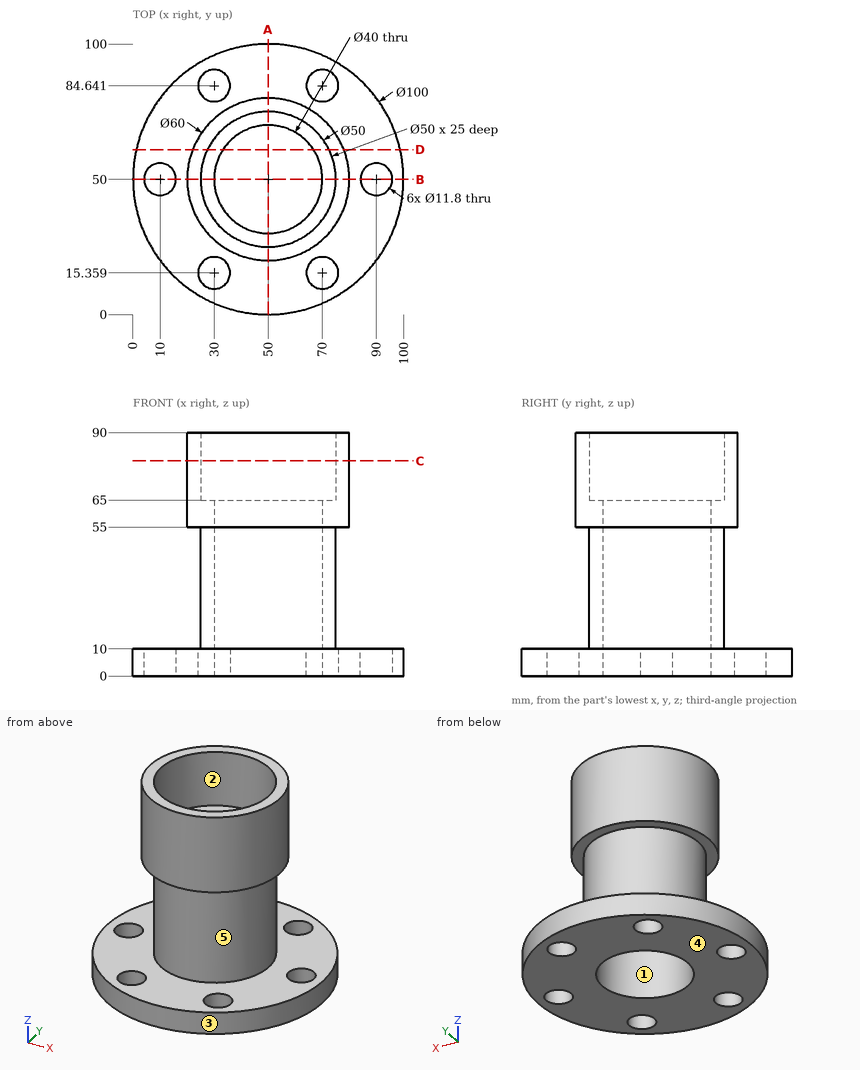
Here's the drawing with two shaded views (mm, measured from the low corner). I have some questions. A direction names the side the tool comes from. Give positions to 0.01 mm unless a question says otherwise; leave off trailing zeros. Loops run counter-clockwise (first coordinate to the right, second up) from the corner with the lowest first, then second, coordinate; pieces in that order, holes last. Notation, with made-up numbers: (72, 10.5) -> (96, 10.5) arc R21 ccw to (96, 32.5) -> close; hole circle Ø6 at (55, 2). An arc over 180 degrees is marked (long way). One line per item, written item: value.
Q1. We'd pull the mould along Z, two halves only. Please class the marked faces 3, 4 and 5: pulls with the +Z half, pulls with the -Z half, needs draft (parallel to the pull), parting line crosses it, or undercut.
Answers follow:
face 3: needs draft
face 4: pulls with the -Z half
face 5: undercut
Q2. Suppose I cut it at C-C on z = 79.5. Please give me the cut outline in (x, y), then the cut area to 3 significant figures.
Answers follow:
outline: circle Ø60 at (50, 50); hole circle Ø50 at (50, 50)
area: 864 mm^2
Q3. On a 3-axis mill with a long thin cutter (end or side, diameter ignored), from which of +Z, -Z, +X, -X, +Y, -Y can I reach the whole of each face in a straight line? I mean the marked faces 1 and 2. Say none if no direction works.
Answers follow:
face 1: +Z, -Z
face 2: +Z
Q4. I'm going to push flat-ended pins straight in: pin 1 Ø1 at (x, z) = (34, 77) entering from -Y; pin 2 Ø13.5 at (x, y) = (70, 84.64) entering from +Z; pin 3 Ø12 at (x, z) = (67.5, 57) entering from +Y; pin 4 Ø3 at (x, y) = (68, 43.5) entering from -Z. Where does each tip first touch, or does it pass through?
Answers follow:
pin 1: y = 24.31
pin 2: z = 10
pin 3: y = 77.71
pin 4: z = 0
Q5. Suppose I cut it at B-B on y = 50. Please give me the cut outline in (x, z), then the cut area to 3 significant figures.
Answers follow:
outline: (0, 0) -> (4.1, 0) -> (4.1, 10) -> (0, 10) -> close; (15.9, 0) -> (30, 0) -> (30, 65) -> (25, 65) -> (25, 90) -> (20, 90) -> (20, 55) -> (25, 55) -> (25, 10) -> (15.9, 10) -> close; (70, 0) -> (84.1, 0) -> (84.1, 10) -> (75, 10) -> (75, 55) -> (80, 55) -> (80, 90) -> (75, 90) -> (75, 65) -> (70, 65) -> close; (95.9, 0) -> (100, 0) -> (100, 10) -> (95.9, 10) -> close
area: 1,260 mm^2
Q6. Suppose I cut it at D-D on y = 61. Please give me the cut outline in (x, z) (3 decimals).
Answers follow:
outline: (1.225, 0) -> (33.297, 0) -> (33.297, 65) -> (27.55, 65) -> (27.55, 90) -> (22.089, 90) -> (22.089, 55) -> (27.55, 55) -> (27.55, 10) -> (1.225, 10) -> close; (66.703, 0) -> (98.775, 0) -> (98.775, 10) -> (72.45, 10) -> (72.45, 55) -> (77.911, 55) -> (77.911, 90) -> (72.45, 90) -> (72.45, 65) -> (66.703, 65) -> close
Q7. Suppose I cut it at A-A on x = 50. Please give me the cut outline in (y, z).
Answers follow:
outline: (0, 0) -> (30, 0) -> (30, 65) -> (25, 65) -> (25, 90) -> (20, 90) -> (20, 55) -> (25, 55) -> (25, 10) -> (0, 10) -> close; (70, 0) -> (100, 0) -> (100, 10) -> (75, 10) -> (75, 55) -> (80, 55) -> (80, 90) -> (75, 90) -> (75, 65) -> (70, 65) -> close
Q8. If I drill on line 1 along Z through (x, y) = (37.5, 27.5); line 2 along X through (y, z) = (50, 32); line 3 along Y through (x, z) = (10, 5.25), over which ranges is the centre line in solid material (lowest first)?
Answers follow:
line 1: 0 to 10, 55 to 90
line 2: 25 to 30, 70 to 75
line 3: 20 to 44.1, 55.9 to 80
